Input: part model. Units: mm. Frame: model coordinates. Face numbers are marked on the shaded views. A direction names the side the tool comes from. Coordinates: 2 decimals unless noted, no trailing zeros. Order: outer loops, then holes, each group sorted by start corner. A loop starts at its lowest first (then second) coordinate and runs counter-clockwise, first axis right, second up. Notation, with made-up numbers: (70.25, 82.25) -> (94.25, 82.25) arc R24 cw to (94.25, 112.25) -> close; hole circle Ø4 at (69, 26.5). An arc over 180 degrees is marked (long way). One line per question, with ' | ' between items.
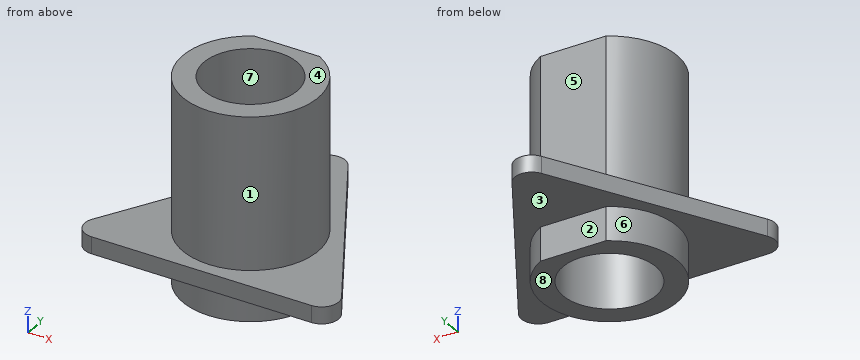
```python
from build123d import *

# Parameters (mm, degrees)
EXTRUDE_1_DEPTH     = 12
EXTRUDE_2_DEPTH     = 1
SKETCH_2_R          = 2.75
CUT_EXTRUDE_1_DEPTH = 100


with BuildPart() as part:
    # 草图1 → 凸台-拉伸1 (new body)
    with BuildSketch(Plane.XY):
        with BuildLine():
            Line((-1.936491673, 3.5), (1.936491673, 3.5))
            ThreePointArc((1.936491673, 3.5), (0, -4), (-1.936491673, 3.5))
        make_face()
    extrude(amount=EXTRUDE_1_DEPTH)

    # 草图3 → 凸台-拉伸2 (add)
    with BuildSketch(Plane.XY.offset(3)):
        with BuildLine():
            Line((-6.495190528, -4.75), (6.495190528, -4.75))
            ThreePointArc((6.495190528, -4.75), (7.361215932, -4.25), (7.361215932, -3.25))
            Line((7.361215932, -3.25), (0.866025404, 8))
            ThreePointArc((0.866025404, 8), (0, 8.5), (-0.866025404, 8))
            Line((-0.866025404, 8), (-7.361215932, -3.25))
            ThreePointArc((-7.361215932, -3.25), (-7.361215932, -4.25), (-6.495190528, -4.75))
        make_face()
    extrude(amount=-EXTRUDE_2_DEPTH)

    # 草图2 → 切除-拉伸1 (cut)
    with BuildSketch(Plane.XY.offset(12)):
        Circle(SKETCH_2_R)
    extrude(amount=-CUT_EXTRUDE_1_DEPTH, mode=Mode.SUBTRACT)


solid = part.part
```
1. Cut plane A-A, the plane y = 0.25. Return loops of the section in (x, z), and give its area (3 significant figures).
Recorded:
outline: (-5.34, 2) -> (-3.99, 2) -> (-3.99, 0) -> (-2.74, 0) -> (-2.74, 12) -> (-3.99, 12) -> (-3.99, 3) -> (-5.34, 3) -> close; (2.74, 0) -> (3.99, 0) -> (3.99, 2) -> (5.34, 2) -> (5.34, 3) -> (3.99, 3) -> (3.99, 12) -> (2.74, 12) -> close | area: 32.8 mm^2
2. Cut plane B-B, the plane x = -2.5. Return loops of the section in (y, z), and give its area (3 significant figures).
Recorded:
outline: (-4.75, 2) -> (-3.12, 2) -> (-3.12, 0) -> (-1.15, 0) -> (-1.15, 12) -> (-3.12, 12) -> (-3.12, 3) -> (-4.75, 3) -> close; (1.15, 0) -> (3.12, 0) -> (3.12, 2) -> (5.17, 2) -> (5.17, 3) -> (3.12, 3) -> (3.12, 12) -> (1.15, 12) -> close | area: 51.1 mm^2
3. Cut plane C-C, the plane z = 2.75. Return loops of the section in (x, y), and give its area (3 significant figures).
Recorded:
outline: (-7.36, -3.25) arc R1 ccw to (-6.5, -4.75) -> (6.5, -4.75) arc R1 ccw to (7.36, -3.25) -> (0.87, 8) arc R1 ccw to (-0.87, 8) -> close; hole circle Ø5.5 at (0, 0) | area: 91.4 mm^2
4. Mould query, pull axis Y, two halves, no side actions, for the marked faces 6, 7 and 8. Classes: released by +Y, released by -Y, zero draft, split by the parting line, or undercut.
Recorded:
face 6: split by the parting line | face 7: undercut | face 8: zero draft
5. Cut plane D-D, the plane y = 5.25. Return loops of the section in (x, z).
Recorded:
outline: (-2.45, 2) -> (2.45, 2) -> (2.45, 3) -> (-2.45, 3) -> close
6. Access query for the marked faces 1, 2, 3, 4 and 5. Directions: +Z, -Z, +X, -X, +Y, -Y. A direction counts if a zero-diameter tool reaches every point of the face in a straight line with its end or side. Return the directions, or none.
Recorded:
face 1: +Z | face 2: -Z, +X, -X, +Y | face 3: -Z | face 4: +Z, +X, -X, +Y, -Y | face 5: +Z, +X, -X, +Y
7. Ray query, line 1 (Y direction, x = 0, z = 7.25); line 2 (Z direction, x = -3.75, y = 2); line 3 (X direction, y = 2, z = 5.5). Return the intervals inside material, ascending. Write a range as [from, to].
Recorded:
line 1: y = [-4, -2.75], [2.75, 3.5] | line 2: z = [2, 3] | line 3: x = [-3.46, -1.89], [1.89, 3.46]
8. Pin query (flat end, axial travel): pin 1 Ø5 at (x, z) = (-0.5, 8) entering from -Y; pin 2 Ø1 at (y, z) = (0.5, 7) entering from -X; pin 3 Ø6 at (x, z) = (-6, 10.5) entering from +Y. Return the tip coordinate at first contact, or that it passes through.
Recorded:
pin 1: stops at y = -4 | pin 2: stops at x = -4 | pin 3: stops at y = 2.65
